Could you check a few things on this model? Use its own coordinates, in mm. Coordinates: 2 decimals unless noted, no trailing zeros. Write each loop counter-clockwise with the first axis right and the second up, starting at its lowest first coordinate (ties: lowest second). Pieces come first, ordered by that corner, then holes. Notation, with made-up numbers: (46.25, -21) - (52.25, -21) arc R23 ccw to (52.25, -6) - close; hole circle Ø9 at (-27.75, 30.5). An arc over 180 degrees is marked (long way). Answer as a JSON object with one key per item and string values. Group by question number.
1) If we section it at B-B (x = 261.5): Write out the boundary of the cut face in (y, z), plus the area to 3 significant figures.
2) If we section it at C-C (z = 16.25): Write out the boundary of the cut face in (x, y).
3) Please list where these lines run through material, in increasing order: line 1 along Y through (x, z) = (308.5, 10); line 2 along Y through (x, z) = (1061, 3).
4) Will these pins go through, and if not, where does the flat tip stop? pin 1 Ø2 at (x, z) = (255.5, 6.5) entering from -Y; pin 2 Ø2 at (x, z) = (412.5, 5) entering from +Y; pin 3 Ø3 at (x, z) = (563.5, 8) entering from -Y; pin 4 Ø9.5 at (x, y) = (954.38, 254.98) entering from -Z.
5) If we section it at A-A (y = 0): Write out the boundary of the cut face in (x, z), plus the area to 3 significant figures.
```python
from build123d import *

# Parameters (mm, degrees)
EXTRUDE_1_DEPTH = 20


with BuildPart() as part:
    # Эскиз1 → Вытянуть-Тонкостенный1 (new body)
    with BuildSketch(Plane.XY):
        with BuildLine():
            ThreePointArc((912.491816875, 238.182711116), (921.250664821, 251.157512727), (907.99238472, 242.833997667))
            ThreePointArc((907.99238472, 242.833997667), (907.709433669, 238.751494744), (904.472489462, 236.247680931))
            Line((904.472489462, 236.247680931), (-4.104867197, 17.011762557))
            ThreePointArc((-4.104867197, 17.011762557), (-17.011762557, -4.104867197), (4.104867197, -17.011762557))
            Line((4.104867197, -17.011762557), (1180.346735421, 266.81048364))
            ThreePointArc((1180.346735421, 266.81048364), (1193.253630781, 287.927113394), (1172.137001027, 300.834008754))
            Line((1172.137001027, 300.834008754), (968.462324862, 251.688160741))
            ThreePointArc((968.462324862, 251.688160741), (964.439737623, 252.440279959), (962.326140621, 255.944505854))
            ThreePointArc((962.326140621, 255.944505854), (946.7309564, 257.30580058), (960.442997448, 249.753130556))
            Line((960.442997448, 249.753130556), (961.20027756, 249.100040338))
            ThreePointArc((961.20027756, 249.100040338), (945.774231381, 257.596794115), (963.318813629, 256.065337549))
            ThreePointArc((963.318813629, 256.065337549), (965.009691231, 253.261956833), (968.227761022, 252.660261458))
            Line((968.227761022, 252.660261458), (1171.902437187, 301.806109471))
            ThreePointArc((1171.902437187, 301.806109471), (1194.225731499, 288.161677234), (1180.581299261, 265.838382922))
            Line((1180.581299261, 265.838382922), (4.339431037, -17.983863275))
            ThreePointArc((4.339431037, -17.983863275), (-17.983863275, -4.339431037), (-4.339431037, 17.983863275))
            Line((-4.339431037, 17.983863275), (904.237925622, 237.219781649))
            ThreePointArc((904.237925622, 237.219781649), (906.827480988, 239.222832699), (907.053841829, 242.488835037))
            ThreePointArc((907.053841829, 242.488835037), (921.969406942, 251.852789481), (912.115703003, 237.256137668))
            Line((912.115703003, 237.256137668), (912.491816875, 238.182711116))
        make_face()
    extrude(amount=EXTRUDE_1_DEPTH)


solid = part.part
```
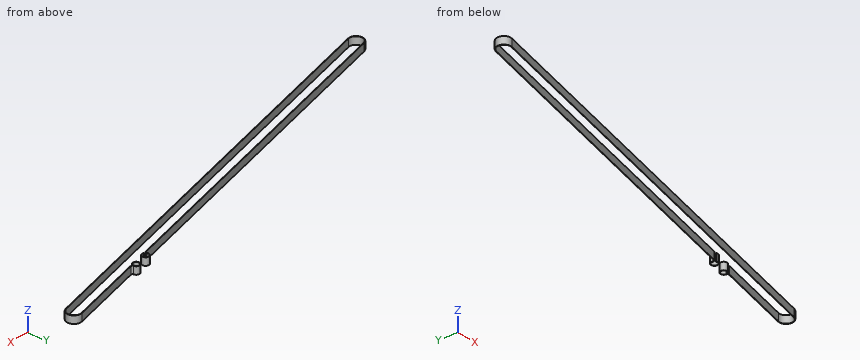
Here are the results:
{
 "1": {"outline": "(44.07, 0) - (45.1, 0) - (45.1, 20) - (44.07, 20) - close; (81.1, 0) - (82.13, 0) - (82.13, 20) - (81.1, 20) - close", "area": "41.1 mm²"},
 "2": {"outline": "(-4.34, 17.98) arc R18.5 ccw to (4.34, -17.98) - (1180.58, 265.84) arc R18.5 ccw to (1171.9, 301.81) - (968.23, 252.66) arc R4 cw to (963.32, 256.07) arc R9 ccw (long way) to (961.2, 249.1) - (960.44, 249.75) arc R8 cw (long way) to (962.33, 255.94) arc R5 ccw to (968.46, 251.69) - (1172.14, 300.83) arc R17.5 cw to (1180.35, 266.81) - (4.1, -17.01) arc R17.5 cw to (-4.1, 17.01) - (904.47, 236.25) arc R5 ccw to (907.99, 242.83) arc R8 cw (long way) to (912.49, 238.18) - (912.12, 237.26) arc R9 ccw (long way) to (907.05, 242.49) arc R4 cw to (904.24, 237.22) - close"},
 "3": {"line 1": "y = 55.41 to 56.44, 92.44 to 93.47", "line 2": "y = 236.98 to 238.01, 274.02 to 275.05"},
 "4": {"pin 1": "stops at y = 42.38", "pin 2": "stops at y = 118.81", "pin 3": "stops at y = 116.58", "pin 4": "passes through"},
 "5": {"outline": "(-18.5, 0) - (-17.5, 0) - (-17.5, 20) - (-18.5, 20) - close; (74.61, 0) - (78.87, 0) - (78.87, 20) - (74.61, 20) - close", "area": "105 mm²"}
}
